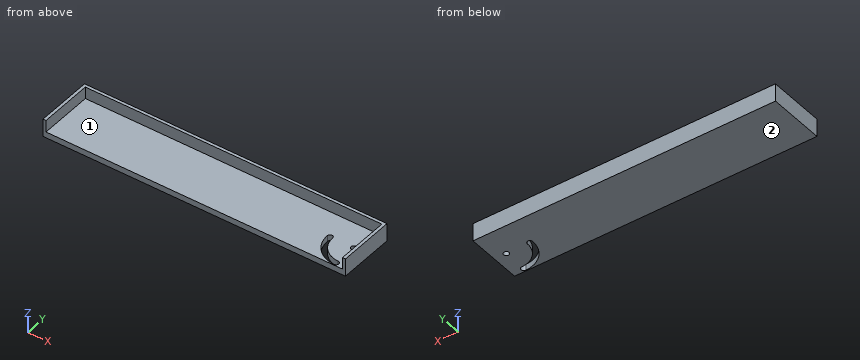
```python
from build123d import *

# Parameters (mm, degrees)
SKETCH1_W           = 510
SKETCH1_H           = 100
SKETCH1_W_2         = 500
SKETCH1_H_2         = 90
BOSS_EXTRUDE1_DEPTH = 20
SKETCH2_W           = 510
SKETCH2_H           = 100
BOSS_EXTRUDE2_DEPTH = 10
SKETCH3_R           = 4.5
CUT_EXTRUDE1_DEPTH  = 1070
SKETCH4_W           = 510
SKETCH4_H           = 5
CUT_EXTRUDE2_DEPTH  = 20


with BuildPart() as part:
    # Sketch1 → Boss-Extrude1 (new body)
    with BuildSketch(Plane.XY):
        with Locations((255, -50)):
            Rectangle(SKETCH1_W, SKETCH1_H)
        with Locations((255, -50)):
            Rectangle(SKETCH1_W_2, SKETCH1_H_2, mode=Mode.SUBTRACT)
    extrude(amount=BOSS_EXTRUDE1_DEPTH)

    # Sketch2 → Boss-Extrude2 (add)
    with BuildSketch(Plane.XY):
        with Locations((255, -50)):
            Rectangle(SKETCH2_W, SKETCH2_H)
    extrude(amount=-BOSS_EXTRUDE2_DEPTH)

    # Sketch3 → Cut-Extrude1 (cut)
    with BuildSketch(Plane.XY):
        with Locations((490, -49)):
            Circle(SKETCH3_R)
        with BuildLine():
            ThreePointArc((490, -93.5), (494.5, -89), (490, -84.5))
            ThreePointArc((490, -84.5), (464.897709268, -74.102290733), (454.5, -49.000000001))
            ThreePointArc((454.5, -49.000000001), (450.000000001, -44.5), (445.5, -49))
            ThreePointArc((445.5, -49), (458.533748237, -80.466251763), (490, -93.5))
        make_face()
    extrude(amount=-CUT_EXTRUDE1_DEPTH, mode=Mode.SUBTRACT)

    # Sketch4 → Cut-Extrude2 (cut, symmetric)
    with BuildSketch(Plane.XY):
        with Locations((255, -97.5)):
            Rectangle(SKETCH4_W, SKETCH4_H)
    extrude(amount=CUT_EXTRUDE2_DEPTH, both=True, mode=Mode.SUBTRACT)


solid = part.part
```
Design review of the part built by this model. Coordinates are the model's own, in mm. Face numbers are marked on the shaded views. Give positions to 0.01 mm unless a question says otherwise; leave off trailing zeros. Order: outer loops, then holes, each group sorted by start corner. A loop starts at its lowest first (then second) coordinate and runs counter-clockwise, first axis right, second up. Notation, with made-up numbers: M 30,24.25 L 52,24.25 A9 cw 52,39.25 Z; hole C 25,46.5 d7. An arc over 180 degrees is marked long. One line per question, with ' | ' between items. Start each with the question number.
Q1. For L1, parallel to Y at x = 490, z = -5.75; L2, parallel to X at y = -44, z = 16.75; L3, parallel to X at y = -45.5, z = -1.5, list the stretches that pass through material, from the lowest coordinate up. Write a range as [from, to].
Q2. We need section C-C (y = -38.5). Write out the cut boundary in (x, z), plus the area to 3 significant figures.
Q3. For pin 1 Ø10 at (x, z) = (346.5, 6) entering from -Y; pin 2 Ø5.5 at (x, y) = (490, -49) entering from -Z; pin 3 Ø8 at (x, y) = (186.5, -85) entering from +Z, all flat-tipped, find the tip position at first contact; note any pin that passes through.
Q4. We need section B-B (y = -89). Write out the cut boundary in (x, z), plus the area to 3 significant figures.
Q5. We need section A-A (x = 450). Write out the cut boundary in (y, z).
Q6. The part is to be moulded in two halves that separate along X. For the marked faces 1 and 2, say which applies: +X half, -X half, draft (parallel to the pull), parting line (faces both ways), or undercut.
Q7. We need section D-D (x = 142.5). Write out the cut boundary in (y, z).
Returned:
1) L1: [-95, -93.5], [-84.5, -53.5], [-44.5, 0] | L2: [0, 5], [505, 510] | L3: [0, 447.17], [452.83, 487.17], [492.83, 510]
2) outline: M 0,-10 L 510,-10 L 510,20 L 505,20 L 505,0 L 5,0 L 5,20 L 0,20 Z | area: 5,300 mm2
3) pin 1: y = -5 | pin 2: through | pin 3: z = 0
4) outline: M 0,-10 L 470.5,-10 L 470.5,0 L 5,0 L 5,20 L 0,20 Z; M 494.5,-10 L 510,-10 L 510,20 L 505,20 L 505,0 L 494.5,0 Z | area: 5,060 mm2
5) outline: M -95,-10 L -68.5,-10 L -68.5,0 L -95,0 Z; M -44.5,-10 L 0,-10 L 0,20 L -5,20 L -5,0 L -44.5,0 Z
6) face 1: undercut | face 2: draft
7) outline: M -95,-10 L 0,-10 L 0,20 L -5,20 L -5,0 L -95,0 Z
